Check sheet for the drawn part. Datum: minimum x, y, z corner. Units: mm. A direction names the side the tool comes from. Coordinates: 2 decimals unless noted, no trailing zeros. Write each loop counter-clockwise with the first axis right and the second up, starting at its lowest first coordinate (ties: lowest second). Pieces come first, ordered by that corner, then holes. Notation, with made-up numbers: M -27.5,66 L 13.5,66 A31 cw 13.5,96 Z; hole C 8,10 d11. An arc over 180 degrees is marked long. Write item = value, one per line. Start each with the question number.
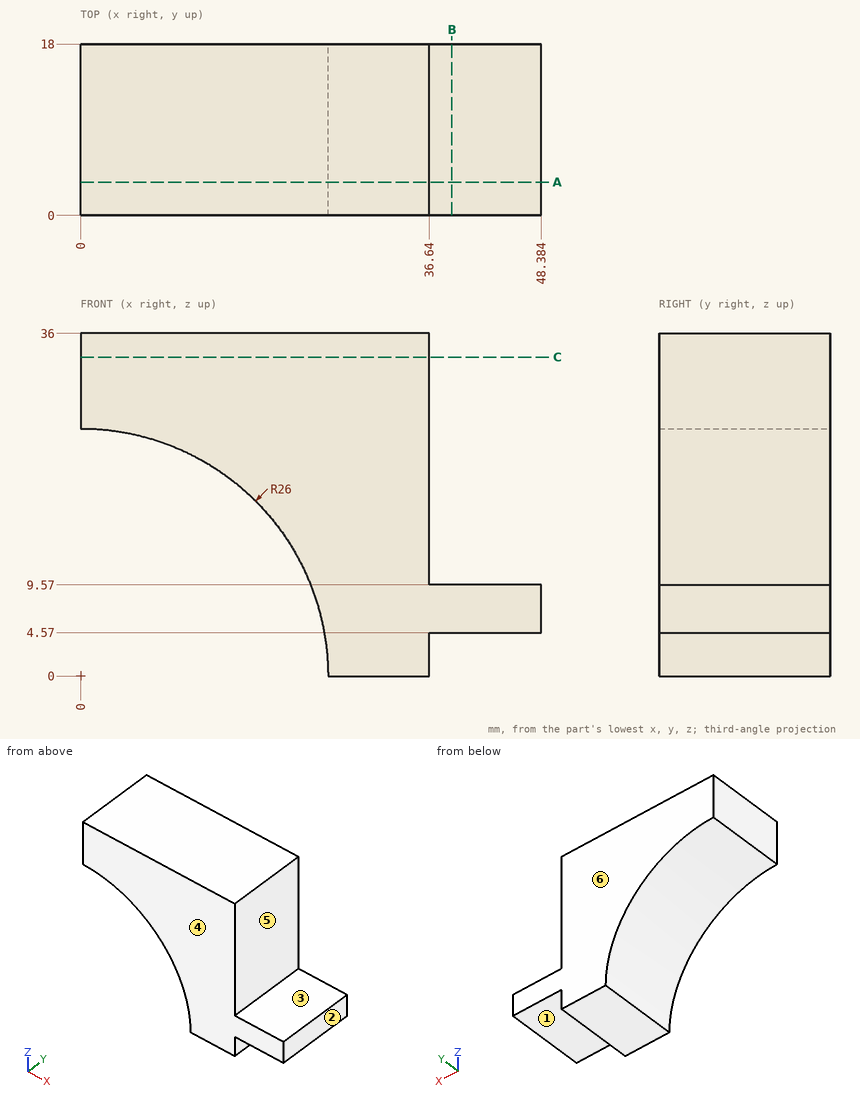
Q1. Set-up check for the marked faces 1, 2 and 3: record each of +Z, -Z, +X, -X, +Y, -Y from which the full face is reachable in a straight line by a thin tool's end or side.
Q2. Draft check along Y on the marked faces 4, 5 and 6. Enter one of: pulls with the +Y half, pulls with the -Y half, needs draft (parallel to the pull), parting line crosses it, or undercut.
Q3. Scan lines: L1, parallel to X at y = 6.5, z = 33.5; L2, parallel to Z at x = 41, y = 5.75; L3, parallel to X at y = 2.75, z = 7. Record each from-to range of solid material in increasing order.
Q4. Cross-section at A-A on y = 3.5. Enter the section's corners in (x, z).
Q5. Gauge pin test, flat ends, axial feed: pin 1 (3.5 mm diameter, centred on x = 40.5, y = 7, fed in from -Z); pin 2 (2 mm diameter, centred on y = 15.5, z = 6.5, fed in from -X); pin 3 (8 mm diameter, centred on y = 14, z = 4, fed in from -X). Record the tip position at first contact, or that the pin passes through.
Q6. Cross-section at B-B on x = 39. Enter the section's corners in (y, z), and give its area (3 significant figures).
Q7. Cross-section at C-C on z = 33.5. Enter the section's corners in (x, y).
Values found:
q1.face_1 = -Z, +X, +Y, -Y
q1.face_2 = +Z, -Z, +X, +Y, -Y
q1.face_3 = +Z, +X, +Y, -Y
q2.face_4 = pulls with the -Y half
q2.face_5 = needs draft
q2.face_6 = pulls with the +Y half
q3.L1 = 0 to 36.64
q3.L2 = 4.57 to 9.57
q3.L3 = 25.04 to 48.38
q4.outline = M 0,26 A26 cw 26,0 L 36.64,0 L 36.64,4.57 L 48.38,4.57 L 48.38,9.57 L 36.64,9.57 L 36.64,36 L 0,36 Z
q5.pin_1 = 4.57
q5.pin_2 = 24.89
q5.pin_3 = 24.74
q6.outline = M 0,4.57 L 18,4.57 L 18,9.57 L 0,9.57 Z
q6.area = 90.0 mm²
q7.outline = M 0,0 L 36.64,0 L 36.64,18 L 0,18 Z
